Can you work these out from the model? Positions are in its coordinate system, mm. Face numbers are marked on the shaded views. A direction names the side the tool comes from. Round coordinates to 2 decimals unless told otherwise and drop trailing zeros. Loops run counter-clockwise (first coordinate to the right, second up) from the corner with the lowest first, then second, coordinate; pieces in that order, holes last. Notation, with made-up numbers: (82.5, 19) -> (122.5, 19) arc R14 cw to (122.5, 40) -> close; hole circle Ø11 at (73, 1.25). An arc over 180 degrees is marked (long way). Answer as a JSON object with one key per item and string values.
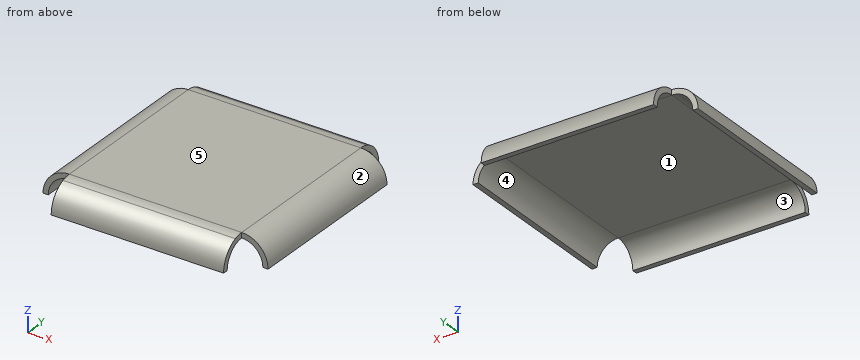
```python
from build123d import *

# Parameters (mm, degrees)
SKETCH1_W                  = 431.8
SKETCH1_H                  = 431.8
BOSS_EXTRUDE1_DEPTH        = 3.175
CONVERT_SOLID2_START       = -431.8
CONVERT_SOLID2_DEPTH       = 431.8
CONVERT_SOLID2_2_DEPTH     = 50.480000066
CONVERT_SOLID2_START_2     = -50.480000066
CONVERT_SOLID2_3_DEPTH     = 50.480000066
CONVERT_SOLID2_START_3     = -381.319999934
CONVERT_SOLID2_4_DEPTH     = 330.839999868
CONVERT_SOLID2_START_4     = -387.436868
CONVERT_SOLID2_5_OUTLINE_W = 330.839999868
CONVERT_SOLID2_5_OUTLINE_H = 6.825
CONVERT_SOLID2_5_DEPTH     = 345.44
CONVERT_SOLID2_START_5     = 50.480000066
CONVERT_SOLID2_6_DEPTH     = 330.839999868


with BuildPart() as part:
    # Sketch1 → Boss-Extrude1 (new body)
    with BuildSketch(Plane.XY):
        with Locations((-215.9, 215.9)):
            Rectangle(SKETCH1_W, SKETCH1_H)
    extrude(amount=BOSS_EXTRUDE1_DEPTH)

    # Convert-Solid2: read off the stored shape, not the designer's step
    # Convert-Solid2 outline → Convert-Solid2 (cut)
    with BuildSketch(Plane.YZ.offset(CONVERT_SOLID2_START)):
        with BuildLine():
            ThreePointArc((32.859915633, 0), (41.528072893, 2.37490942), (50.480000066, 3.175))
            Line((50.480000066, 3.175), (0, 3.175))
            Line((0, 3.175), (0, 0))
            Line((0, 0), (32.859915633, 0))
        make_face()
        with BuildLine():
            Line((431.8, 3.175), (381.319999934, 3.175))
            ThreePointArc((381.319999934, 3.175), (390.271927107, 2.37490942), (398.940084367, 0))
            Line((398.940084367, 0), (431.8, 0))
            Line((431.8, 0), (431.8, 3.175))
        make_face()
    extrude(amount=CONVERT_SOLID2_DEPTH, mode=Mode.SUBTRACT)

    # Convert-Solid2 2 outline → Convert-Solid2 2 (cut)
    with BuildSketch(Plane.YZ.offset(CONVERT_SOLID2_START)):
        with BuildLine():
            Line((32.859915633, 0), (398.940084367, 0))
            ThreePointArc((398.940084367, 0), (390.271927107, 2.37490942), (381.319999934, 3.175))
            Line((381.319999934, 3.175), (50.480000066, 3.175))
            ThreePointArc((50.480000066, 3.175), (41.528072893, 2.37490942), (32.859915633, 0))
        make_face()
    extrude(amount=CONVERT_SOLID2_2_DEPTH, mode=Mode.SUBTRACT)

    # Convert-Solid2 3 outline → Convert-Solid2 3 (cut)
    with BuildSketch(Plane.YZ.offset(CONVERT_SOLID2_START_2)):
        with BuildLine():
            Line((32.859915633, 0), (398.940084367, 0))
            ThreePointArc((398.940084367, 0), (390.271927107, 2.37490942), (381.319999934, 3.175))
            Line((381.319999934, 3.175), (50.480000066, 3.175))
            ThreePointArc((50.480000066, 3.175), (41.528072893, 2.37490942), (32.859915633, 0))
        make_face()
    extrude(amount=CONVERT_SOLID2_3_DEPTH, mode=Mode.SUBTRACT)

    # Convert-Solid2 4 outline → Convert-Solid2 4 (add)
    with BuildSketch(Plane.YZ.offset(CONVERT_SOLID2_START_3)):
        with BuildLine():
            ThreePointArc((10, -47.305000066), (21.856317517, -18.681317517), (50.480000066, -6.825))
            Line((50.480000066, -6.825), (381.319999934, -6.825))
            ThreePointArc((381.319999934, -6.825), (409.943682483, -18.681317517), (421.8, -47.305000066))
            Line((421.8, -47.305000066), (431.8, -47.305000066))
            ThreePointArc((431.8, -47.305000066), (422.778969229, -18.505967588), (398.940084367, 0))
            Line((398.940084367, 0), (32.859915633, 0))
            ThreePointArc((32.859915633, 0), (9.021030771, -18.505967588), (0, -47.305000066))
            Line((0, -47.305000066), (10, -47.305000066))
        make_face()
    extrude(amount=CONVERT_SOLID2_4_DEPTH)

    # Convert-Solid2 5 outline → Convert-Solid2 5 (add)
    with BuildSketch(Plane.YZ.offset(CONVERT_SOLID2_START_4)):
        with Locations((215.9, -3.4125)):
            Rectangle(CONVERT_SOLID2_5_OUTLINE_W, CONVERT_SOLID2_5_OUTLINE_H)
    extrude(amount=CONVERT_SOLID2_5_DEPTH)

    # Convert-Solid2 6 outline → Convert-Solid2 6 (add)
    with BuildSketch(Plane(origin=(0, 0, 0), x_dir=(1, 0, 0), z_dir=(0, 1, 0)).offset(CONVERT_SOLID2_START_5)):
        with BuildLine():
            ThreePointArc((-50.480000066, -3.175), (-14.785249705, 11.610249705), (0, 47.305000066))
            Line((0, 47.305000066), (-10, 47.305000066))
            ThreePointArc((-10, 47.305000066), (-21.856317517, 18.681317517), (-50.480000066, 6.825))
            Line((-50.480000066, 6.825), (-50.480000066, 0))
            Line((-50.480000066, 0), (-50.480000066, -3.175))
        make_face()
        with BuildLine():
            ThreePointArc((-381.319999934, 6.825), (-409.943682483, 18.681317517), (-421.8, 47.305000066))
            Line((-421.8, 47.305000066), (-431.8, 47.305000066))
            ThreePointArc((-431.8, 47.305000066), (-417.014750295, 11.610249705), (-381.319999934, -3.175))
            Line((-381.319999934, -3.175), (-381.319999934, 0))
            Line((-381.319999934, 0), (-381.319999934, 6.825))
        make_face()
    extrude(amount=CONVERT_SOLID2_6_DEPTH)


solid = part.part
```
Q1. I want a section at C-C, the plane y = 262.5. Write out the boundary of the cut face in (x, z) (3 decimals), then the cut area to 3 significant figures.
Determined:
{"outline": "(-431.8, -47.305) -> (-421.8, -47.305) arc R40.48 cw to (-381.32, -6.825) -> (-50.48, -6.825) arc R40.48 cw to (-10, -47.305) -> (0, -47.305) arc R50.48 ccw to (-50.48, 3.175) -> (-381.32, 3.175) arc R50.48 ccw to start", "area": "4,740 mm²"}
Q2. On a 3-axis mill with a long thin cutter (end or side, diameter ignored), from which of +Z, -Z, +X, -X, +Y, -Y can I reach the whole of each face in a straight line? I mean the marked faces 3, 4 and 5. Say none if no direction works.
Determined:
{"face 3": "-Z, +X, -X", "face 4": "-Z, +Y, -Y", "face 5": "+Z, +X, -X, +Y, -Y"}
Q3. If I drill on L1, parallel to Z at x = -303.5, y = 234 (3 decimals); L2, parallel to X at y = 341, z = -44; L3, parallel to Y at x = -293.5, z = -13, over which ranges is the centre line in solid material (lowest first)? Write a range as [from, to].
Determined:
{"L1": "[-6.825, 3.175]", "L2": "[-431.69, -421.66], [-10.14, -0.11]", "L3": "[13.45, 28.99], [402.81, 418.35]"}
Q4. I want a section at A-A, the plane z = -17. Write out the boundary of the cut face in (x, y), then the cut area to 3 significant figures.
Determined:
{"outline": "(-421.69, 50.48) -> (-408.16, 50.48) -> (-408.16, 381.32) -> (-421.69, 381.32) -> close; (-381.32, 10.11) -> (-50.48, 10.11) -> (-50.48, 23.64) -> (-381.32, 23.64) -> close; (-381.32, 408.16) -> (-50.48, 408.16) -> (-50.48, 421.69) -> (-381.32, 421.69) -> close; (-23.64, 50.48) -> (-10.11, 50.48) -> (-10.11, 381.32) -> (-23.64, 381.32) -> close", "area": "17,900 mm²"}
Q5. I want a section at B-B, the plane x = -369.5. Write out the boundary of the cut face in (y, z) (3 decimals).
Determined:
{"outline": "(0, -47.305) -> (10, -47.305) arc R40.48 cw to (50.48, -6.825) -> (381.32, -6.825) arc R40.48 cw to (421.8, -47.305) -> (431.8, -47.305) arc R50.48 ccw to (381.32, 3.175) -> (50.48, 3.175) arc R50.48 ccw to start"}
Q6. We'd pull the mould along Y, two halves only. Please class the marked faces 1 and 2: pulls with the +Y half, pulls with the -Y half, needs draft (parallel to the pull), parting line crosses it, or undercut.
Determined:
{"face 1": "undercut", "face 2": "needs draft"}
Q7. I want a section at D-D, the plane z = -40.5. Write out the boundary of the cut face in (x, y), then the cut area to 3 significant figures.
Determined:
{"outline": "(-431.34, 50.48) -> (-421.22, 50.48) -> (-421.22, 381.32) -> (-431.34, 381.32) -> close; (-381.32, 0.46) -> (-50.48, 0.46) -> (-50.48, 10.58) -> (-381.32, 10.58) -> close; (-381.32, 421.22) -> (-50.48, 421.22) -> (-50.48, 431.34) -> (-381.32, 431.34) -> close; (-10.58, 50.48) -> (-0.46, 50.48) -> (-0.46, 381.32) -> (-10.58, 381.32) -> close", "area": "13,400 mm²"}
Q8. I'm going to push flat-ended pins straight in: pin 1 (12 mm diameter, centred on x = -349.5, y = 230, fed in from -Z) (3 decimals); pin 2 (5 mm diameter, centred on x = -45.5, y = 387.5, fed in from -Z); pin 3 (4 mm diameter, centred on x = -383.5, y = 229.5, fed in from -Z); pin 4 (5 mm diameter, centred on y = 112.5, z = -20.5, fed in from +X). Where does each tip first touch, or does it pass through?
Determined:
{"pin 1": "z = -6.825", "pin 2": "through", "pin 3": "z = -7.04", "pin 4": "x = -6.24"}
